The drawing under review shows one solid part. Ordinate dimensions are in mm from its lowest x, y, z. A direction names the side the tool comes from. Coordinates: 2 decimals unless noted, no trailing zeros. Write each loop counter-clockwise with the first axis right and the second up, starting at its lowest first coordinate (ties: lowest second). Pieces come first, ordered by that corner, then holes. Notation, with made-up numbers: (74.25, 15.5) - (132.25, 15.5) arc R9 cw to (132.25, 29.5) - close; hole circle Ø11 at (-20.5, -39.5). An arc over 180 degrees is marked (long way). Use a Markdown table: item, result.
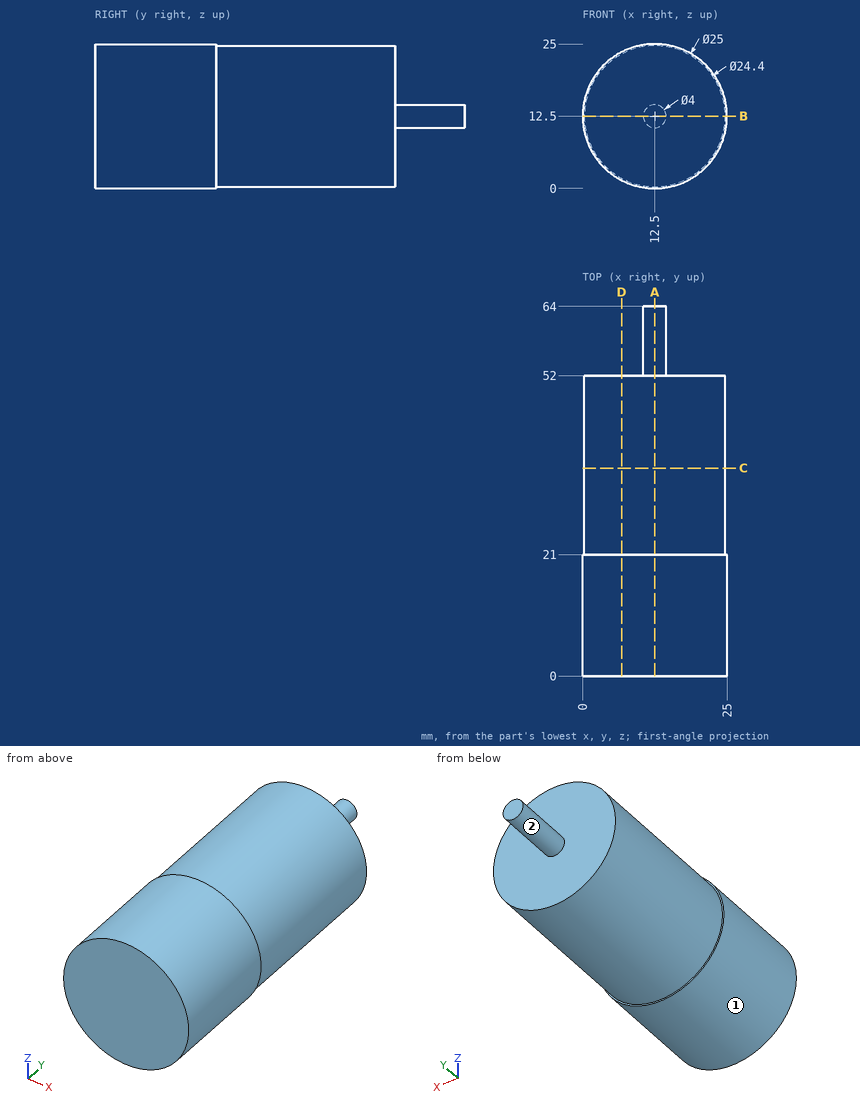
(1) Take a section at C-C on y = 36. Write out the cut boundary in (x, z), and give its area (3 significant figures).
Determined:
| item | result |
|---|---|
| outline | circle Ø24.4 at (12.5, 12.5) |
| area | 468 mm2 |
(2) Take a section at A-A on x = 12.5. Write out the cut boundary in (y, z).
Determined:
| item | result |
|---|---|
| outline | (0, 0) - (21, 0) - (21, 0.3) - (52, 0.3) - (52, 10.5) - (64, 10.5) - (64, 14.5) - (52, 14.5) - (52, 24.7) - (21, 24.7) - (21, 25) - (0, 25) - close |
(3) Machinability: for the marked faces 1 and 2, which of the approach directions +Z, -Z, +X, -X, +Y, -Y give a long, thin tool a straight path to every point of the face, cutting with its end or side? Answer none if there is none.
Determined:
| item | result |
|---|---|
| face 1 | +Y, -Y |
| face 2 | +Y |
(4) Take a section at D-D on x = 6.75. Write out the cut boundary in (y, z).
Determined:
| item | result |
|---|---|
| outline | (0, 1.4) - (21, 1.4) - (21, 1.74) - (52, 1.74) - (52, 23.26) - (21, 23.26) - (21, 23.6) - (0, 23.6) - close |
(5) For pin 1 (2 mm diameter, centred on x = 15.5, z = 13.5, fed in from -Y); pin 2 (10 mm diameter, centred on y = 55.5, z = 13, fed in from +X); pin 3 (5 mm diameter, centred on x = 21, z = 20.5, fed in from +Y); pin 4 (3 mm diameter, centred on y = 41.5, z = 10.5, fed in from -X), all flat-tipped, find the tip position at first contact; note any pin that passes through.
Determined:
| item | result |
|---|---|
| pin 1 | y = 0 |
| pin 2 | x = 24.7 |
| pin 3 | y = 52 |
| pin 4 | x = 0.31 |
(6) For L1, parallel to Y at x = 4.25, z = 5.5; L2, parallel to Z at x = 12.5, y = 54; L3, parallel to Y at x = 8, z = 24, list the stretches that pass through material, from the lowest coordinate up. Write a range as from..to.
Determined:
| item | result |
|---|---|
| L1 | 0..52 |
| L2 | 10.5..14.5 |
| L3 | 0..21 |
(7) Take a section at B-B on z = 12.5. Write out the cut boundary in (x, y).
Determined:
| item | result |
|---|---|
| outline | (0, 0) - (25, 0) - (25, 21) - (24.7, 21) - (24.7, 52) - (14.5, 52) - (14.5, 64) - (10.5, 64) - (10.5, 52) - (0.3, 52) - (0.3, 21) - (0, 21) - close |
